Input: dimensioned drawing with shaded views. Units: mm. Origin: part minimum x, y, z. Give positions to 0.01 mm unless a question says otherwise; leave off trailing zeros. Loops run counter-clockwise (first coordinate to the right, second up) from the corner with the lowest first, then second, coordinate; pieces in that order, holes last. Notation, with made-up numbers: (-2.75, -11) -> (35.25, -11) arc R18 ccw to (35.25, 23) -> close; hole circle Ø10 at (-0.75, 88.5). An arc over 180 degrees is marked (long way). One line per question, with ' | ' between items. Start each with the question number.
Item 1: Section A-A on z = 19. Return loops of the section in (x, y).
Item 2: Section C-C on y = 1.7. Return loops of the section in (x, z) (1 decimal).
Item 3: Section B-B on x = 38.5. Return loops of the section in (y, z) (1 decimal), then the cut area to 3 significant figures.
Item 4: Material intervals for line 1 along Z through (x, y) = (8.5, 1.05) (1 decimal); line 2 along X through (y, z) = (2.15, 19.5); line 3 along X through (y, z) = (2.3, 32.5), sorted ascending. Write a range as [from, to].
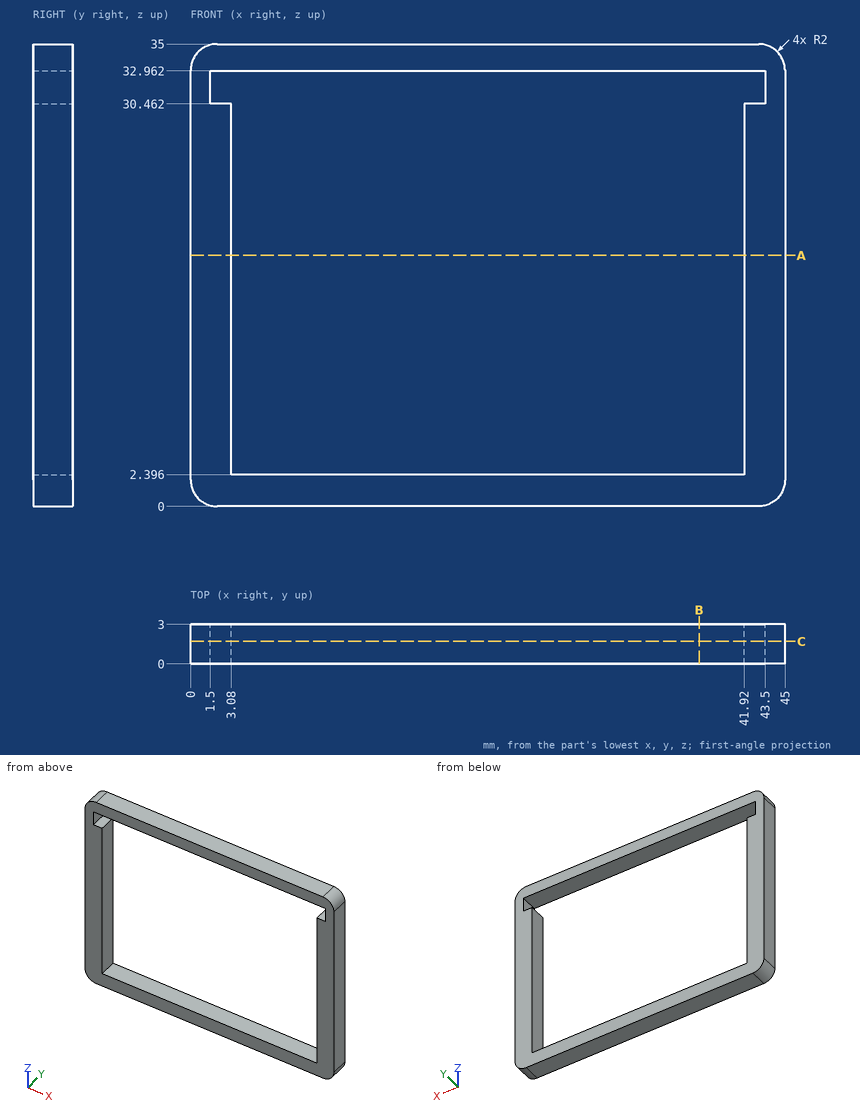
Result sheet:
1) outline: (0, 0) -> (3.08, 0) -> (3.08, 3) -> (0, 3) -> close; (41.92, 0) -> (45, 0) -> (45, 3) -> (41.92, 3) -> close
2) outline: (0, 2) arc R2 ccw to (2, 0) -> (43, 0) arc R2 ccw to (45, 2) -> (45, 33) arc R2 ccw to (43, 35) -> (2, 35) arc R2 ccw to (0, 33) -> close; hole (1.5, 30.5) -> (3.1, 30.5) -> (3.1, 2.4) -> (41.9, 2.4) -> (41.9, 30.5) -> (43.5, 30.5) -> (43.5, 33) -> (1.5, 33) -> close
3) outline: (0, 0) -> (3, 0) -> (3, 2.4) -> (0, 2.4) -> close; (0, 33) -> (3, 33) -> (3, 35) -> (0, 35) -> close | area: 13.3 mm²
4) line 1: z = [0, 2.4], [33, 35] | line 2: x = [0, 3.08], [41.92, 45] | line 3: x = [0, 1.5], [43.5, 45]
